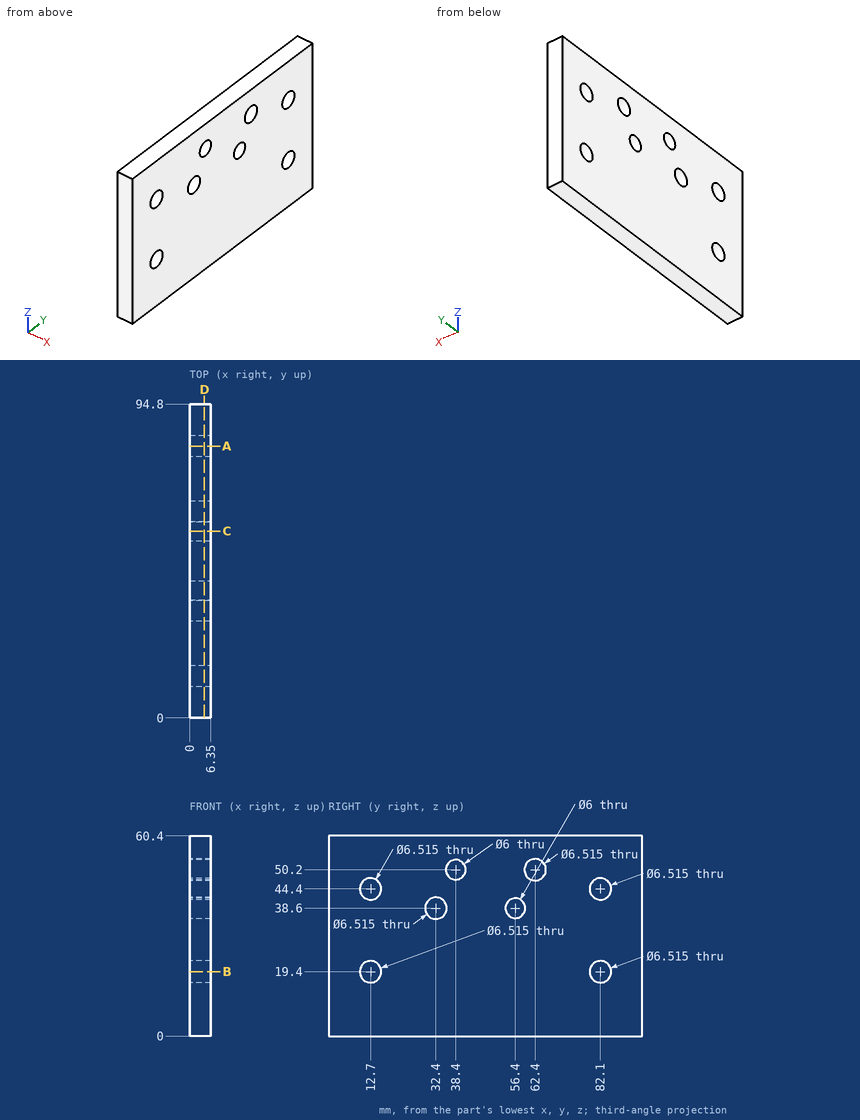
Input: dimensioned drawing with shaded views. Units: mm. Origin: part minimum x, y, z. Round coordinates to 2 decimals unless told otherwise and drop trailing zeros. Order: outer loops, then holes, each group sorted by start corner. A loop starts at its lowest first (then second) coordinate and runs counter-clockwise, first axis right, second up. Notation, with made-up numbers: (5, -6) -> (38, -6) arc R24 ccw to (38, 26) -> close; hole circle Ø4 at (84.25, 5.25). An arc over 180 degrees is marked (long way). One line per item, written item: value. Start each with the question number.
Q1. Section query B-B (z = 19.4). Return the cut outline in (x, y), plus the area to 3 significant figures.
Q2. Section query A-A (y = 82.1). Return the cut outline in (x, z), plus the area to 3 significant figures.
Q3. Section query D-D (x = 4.5). Give the number of separate pieces and of enclosed holes in the cut face, plus the area to 3 significant figures.
Q4. Section query C-C (y = 56.4). Return the cut outline in (x, z), plus the area to 3 significant figures.
Q5. Material intervals for probe 1 along Z at (x, y) = (1.75, 12.7); probe 2 along Y at (x, z) = (0.5, 40); probe 3 along Y at (x, z) = (5.25, 17), sorted ascending.
Findings below:
1. outline: (0, 0) -> (6.35, 0) -> (6.35, 9.44) -> (0, 9.44) -> close; (0, 15.96) -> (6.35, 15.96) -> (6.35, 78.84) -> (0, 78.84) -> close; (0, 85.36) -> (6.35, 85.36) -> (6.35, 94.8) -> (0, 94.8) -> close
1. area: 519 mm²
2. outline: (0, 0) -> (6.35, 0) -> (6.35, 16.14) -> (0, 16.14) -> close; (0, 22.66) -> (6.35, 22.66) -> (6.35, 41.14) -> (0, 41.14) -> close; (0, 47.66) -> (6.35, 47.66) -> (6.35, 60.4) -> (0, 60.4) -> close
2. area: 301 mm²
3. separate pieces: 1
3. enclosed holes: 8
3. area: 5,470 mm²
4. outline: (0, 0) -> (6.35, 0) -> (6.35, 35.6) -> (0, 35.6) -> close; (0, 41.6) -> (6.35, 41.6) -> (6.35, 60.4) -> (0, 60.4) -> close
4. area: 345 mm²
5. probe 1: 0 to 16.14, 22.66 to 41.14, 47.66 to 60.4
5. probe 2: 0 to 29.46, 35.34 to 53.75, 59.05 to 94.8
5. probe 3: 0 to 10.5, 14.9 to 79.9, 84.3 to 94.8
